For this review, take the finished solid that the model builds, in its own axes (mm). Face numbers are marked on the shaded views. Give positions to 0.01 mm unless a question says otherwise; leave off trailing zeros. Loops run counter-clockwise (first coordinate to the right, second up) from the corner with the lowest first, then second, coordinate; pieces in that order, holes last. Notation, with made-up numbers: (-21, 45.5) -> (2, 45.5) arc R25 cw to (2, 68.5) -> close; hole circle Ø7 at (43, -38). An arc over 180 degrees is marked (long way). Answer as CSV lines item,"result". Start each with the question number.
Item 1: Add section A-A on z = 11.5. State the section outline as (x, y) points.
Item 2: Add section C-C on x = 2.5. State the section outline as (y, z) points.
Item 3: Clearance check with flat-ended pins moving along their axes: P1, Ø4, axis at y = -5, z = 9.5, coming from the +X side; P2, Ø3, axis at x = 16, y = -5, coming from the +Z side; P3, Ø3.5, axis at x = 10, y = -5, coming from the -Z side. State where each tip first meets the part, or that it passes through.
Item 4: The part is to be moulded in two halves that separate along Z. For the marked faces 1 and 2, say which applies: +Z half, -Z half, draft (parallel to the pull), parting line (faces both ways), or undercut.
Item 5: For L1, parallel to Z at x = 11, y = -0.8; L2, parallel to Z at x = 5.75, y = -6.25; L3, parallel to Y at x = 19, z = 20.5, list the stretches that pass through material, from the lowest coordinate up. Write a range as from..to.
Item 6: Add section D-D on y = -2.5. State the section outline as (x, z) points.
Item 7: Add section B-B on x = 11. State how many separate pieces and enclosed holes the cut face has, plus the area to 3 significant figures.
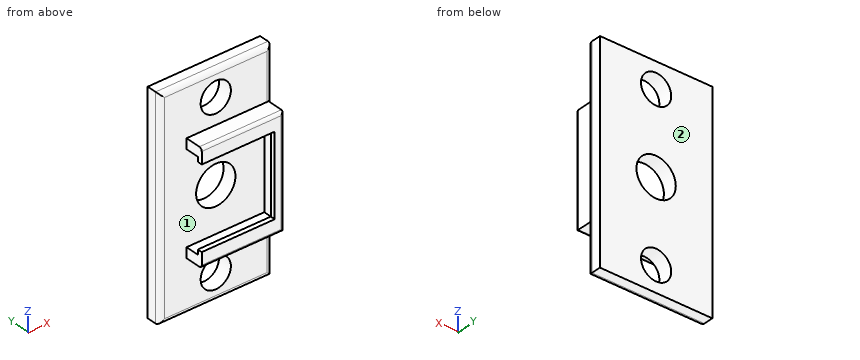
```python
from build123d import *

# Parameters (mm, degrees)
F1_DEPTH      = 3
F2_DEPTH      = 6.85
F6_DEPTH      = 3
F3_W          = 16.2
F3_H          = 1
F7_DEPTH      = 1
F5_W          = 16.2
F5_H          = 1
F8_DEPTH      = 1
F4_W          = 1
F4_H          = 18.8
F9_DEPTH      = 1
F10_D         = 8.2
F0_W          = 23.4142135624
F0_H          = 44.4142135624
F11_DEPTH     = 3
F12_T1_DEPTH  = 28.4142135624
F12_T3_DEPTH  = 49.4142135624
F12_T8_DEPTH  = 49.4142135624
F12_T14_DEPTH = 49.4142135624
F12_T20_DEPTH = 49.4142135624
F12_T27_DEPTH = 49.4142135624
F12_T33_DEPTH = 49.4142135624
F13_R         = 0.6
F14_D         = 6.3


# Not quite as in the source:
# - a fillet or chamfer that OpenCascade refuses, or shapes differently, is made with other operations: its cross-section is extruded or revolved along the edge and cut away or added
# - a feature names something its author has since deleted; it is built from what else it names


with BuildPart() as f1:
    # F0 (on Front) → F1 (new body)
    with BuildSketch(Plane.XZ):
        Polygon((0.9, 2.1), (4.9, 2.1), (21.1, 2.1), (21.1, 20.9), (4.9, 20.9), (0.9, 20.9), align=None)
        Polygon((0, 23), (0, 0), (4.9, 0), (4.9, 2.1), (0.9, 2.1), (0.9, 20.9), (4.9, 20.9), (4.9, 23), align=None)
        Polygon((4.9, 2.1), (4.9, 0), (22, 0), (22, 23), (4.9, 23), (4.9, 20.9), (21.1, 20.9), (21.1, 2.1), align=None)
    extrude(amount=F1_DEPTH)

    # F0 (on Front) → F2 (join)
    with BuildSketch(Plane.XZ):
        Polygon((4.9, 2.1), (4.9, 0), (22, 0), (22, 23), (4.9, 23), (4.9, 20.9), (21.1, 20.9), (21.1, 2.1), align=None)
    extrude(amount=F2_DEPTH)

    # F0 (on Front) → F6 (join)
    with BuildSketch(Plane.XZ):
        Polygon((0, 23), (0, 0), (4.9, 0), (4.9, 2.1), (0.9, 2.1), (0.9, 20.9), (4.9, 20.9), (4.9, 23), align=None)
    extrude(amount=F6_DEPTH)

    # F3 (on face) → F7 (join)
    with BuildSketch(Plane(origin=(0, 0, 20.9), x_dir=(1, 0, 0), z_dir=(0, 0, -1))):
        with Locations((13, 6.35)):
            Rectangle(F3_W, F3_H)
    extrude(amount=F7_DEPTH)

    # F5 (on face) → F8 (join)
    with BuildSketch(Plane.XY.offset(2.1)):
        with Locations((13, -6.35)):
            Rectangle(F5_W, F5_H)
    extrude(amount=F8_DEPTH)

    # F4 (on face) → F9 (join)
    with BuildSketch(Plane(origin=(21.1, 0, 0), x_dir=(0, -1, 0), z_dir=(-1, 0, 0))):
        with Locations((6.35, 11.5)):
            Rectangle(F4_W, F4_H)
    extrude(amount=F9_DEPTH)

    # F10 (through all)
    with Locations(Plane(origin=(0, 0, 0), x_dir=(1, 0, 0), z_dir=(0, 1, 0))):
        with Locations((11, -11.5)):
            Hole(F10_D / 2)

    # F0 (on Front) → F11 (join)
    with BuildSketch(Plane.XZ):
        with Locations((11, 11.5)):
            Rectangle(F0_W, F0_H)
        Polygon((4.9, 0), (0, 0), (0, 23), (4.9, 23), (22, 23), (22, 0), align=None, mode=Mode.SUBTRACT)
    extrude(amount=F11_DEPTH)

    # F12: fillet of radius 1 on 4 edges, made by hand

    # F12_s2 → F12_t1 (cut)
    with BuildSketch(Plane.YZ.offset(-3.2071067812)):
        with BuildLine():
            ThreePointArc((-3, -9.7071067812), (-2.7071067812, -10.4142135624), (-2, -10.7071067812))
            Line((-2, -10.7071067812), (-3, -10.7071067812))
            Line((-3, -10.7071067812), (-3, -9.7071067812))
        make_face()
        with BuildLine():
            ThreePointArc((-3, 32.7071067812), (-2.7071067812, 33.4142135624), (-2, 33.7071067812))
            Line((-2, 33.7071067812), (-3, 33.7071067812))
            Line((-3, 33.7071067812), (-3, 32.7071067812))
        make_face()
    extrude(amount=F12_T1_DEPTH, mode=Mode.SUBTRACT)

    # F12_s4 → F12_t3 (cut)
    with BuildSketch(Plane.XY.offset(-13.2071067812)):
        with BuildLine():
            ThreePointArc((0.2928932188, -3), (-0.4142135624, -2.7071067812), (-0.7071067812, -2))
            Line((-0.7071067812, -2), (-0.7071067812, -3))
            Line((-0.7071067812, -3), (0.2928932188, -3))
        make_face()
    extrude(amount=F12_T3_DEPTH, mode=Mode.SUBTRACT)


with BuildPart() as f12_tool6:
    # F12_s7 → F12_t8 (new body)
    with BuildSketch(Plane.XY.offset(-13.2071067812)):
        with BuildLine():
            ThreePointArc((21.7071067812, -3), (22.4142135624, -2.7071067812), (22.7071067812, -2))
            Line((22.7071067812, -2), (22.7071067812, -3))
            Line((22.7071067812, -3), (21.7071067812, -3))
        make_face()
    extrude(amount=F12_T8_DEPTH)

    split(bisect_by=Plane.XY, keep=Keep.BOTTOM)

    split(bisect_by=Plane.YZ.offset(22), keep=Keep.BOTTOM)


with BuildPart() as f1_1:
    add(f1.part)

    # F12_t5: cut F12_tool6
    add(f12_tool6.part, mode=Mode.SUBTRACT)


with BuildPart() as f12_tool12:
    # F12_s13 → F12_t14 (new body)
    with BuildSketch(Plane.XY.offset(-13.2071067812)):
        with BuildLine():
            ThreePointArc((21.7071067812, -3), (22.4142135624, -2.7071067812), (22.7071067812, -2))
            Line((22.7071067812, -2), (22.7071067812, -3))
            Line((22.7071067812, -3), (21.7071067812, -3))
        make_face()
    extrude(amount=F12_T14_DEPTH)

    split(bisect_by=Plane.XY, keep=Keep.BOTTOM)

    split(bisect_by=Plane.YZ.offset(22), keep=Keep.TOP)


with BuildPart() as f1_2:
    add(f1_1.part)

    # F12_t11: cut F12_tool12
    add(f12_tool12.part, mode=Mode.SUBTRACT)


with BuildPart() as f12_tool18:
    # F12_s19 → F12_t20 (new body)
    with BuildSketch(Plane.XY.offset(-13.2071067812)):
        with BuildLine():
            ThreePointArc((21.7071067812, -3), (22.4142135624, -2.7071067812), (22.7071067812, -2))
            Line((22.7071067812, -2), (22.7071067812, -3))
            Line((22.7071067812, -3), (21.7071067812, -3))
        make_face()
    extrude(amount=F12_T20_DEPTH)

    split(bisect_by=Plane.XY.offset(23), keep=Keep.BOTTOM)

    split(bisect_by=Plane.XY, keep=Keep.TOP)

    split(bisect_by=Plane.YZ.offset(22), keep=Keep.TOP)


with BuildPart() as f1_3:
    add(f1_2.part)

    # F12_t17: cut F12_tool18
    add(f12_tool18.part, mode=Mode.SUBTRACT)


with BuildPart() as f12_tool25:
    # F12_s26 → F12_t27 (new body)
    with BuildSketch(Plane.XY.offset(-13.2071067812)):
        with BuildLine():
            ThreePointArc((21.7071067812, -3), (22.4142135624, -2.7071067812), (22.7071067812, -2))
            Line((22.7071067812, -2), (22.7071067812, -3))
            Line((22.7071067812, -3), (21.7071067812, -3))
        make_face()
    extrude(amount=F12_T27_DEPTH)

    split(bisect_by=Plane.XY.offset(23), keep=Keep.TOP)

    split(bisect_by=Plane.YZ.offset(22), keep=Keep.BOTTOM)


with BuildPart() as f1_4:
    add(f1_3.part)

    # F12_t24: cut F12_tool25
    add(f12_tool25.part, mode=Mode.SUBTRACT)


with BuildPart() as f12_tool31:
    # F12_s32 → F12_t33 (new body)
    with BuildSketch(Plane.XY.offset(-13.2071067812)):
        with BuildLine():
            ThreePointArc((21.7071067812, -3), (22.4142135624, -2.7071067812), (22.7071067812, -2))
            Line((22.7071067812, -2), (22.7071067812, -3))
            Line((22.7071067812, -3), (21.7071067812, -3))
        make_face()
    extrude(amount=F12_T33_DEPTH)

    split(bisect_by=Plane.XY.offset(23), keep=Keep.TOP)

    split(bisect_by=Plane.YZ.offset(22), keep=Keep.TOP)


with BuildPart() as f1_5:
    add(f1_4.part)

    # F12_t30: cut F12_tool31
    add(f12_tool31.part, mode=Mode.SUBTRACT)

    # F13
    f13_edges = [f1_5.edges().sort_by_distance(p)[0] for p in [
        (22, -6.85, 11.5),
        (13.45, -6.85, 0),
        (13.45, -6.85, 23),
    ]]
    fillet(f13_edges, radius=F13_R)

    # F14 (through all)
    with Locations(Plane(origin=(0, 0, 0), x_dir=(1, 0, 0), z_dir=(0, 1, 0))):
        with Locations((11, -28.3535533906), (11, 5.3535533906)):
            Hole(F14_D / 2)


solid = f1_5.part
```
Computed values:
1,outline,"(-0.71, -2) arc R1 ccw to (0.29, -3) -> (6.9, -3) -> (6.9, 0) -> (-0.71, 0) -> close; (15.1, -3) -> (21.1, -3) -> (21.1, -5.85) -> (20.1, -5.85) -> (20.1, -6.85) -> (21.4, -6.85) arc R0.6 ccw to (22, -6.25) -> (22, -2.96) arc R1 ccw to (22.71, -2) -> (22.71, 0) -> (15.1, 0) -> close"
2,outline,"(-3, -9.71) arc R1 ccw to (-2, -10.71) -> (0, -10.71) -> (0, 33.71) -> (-2, 33.71) arc R1 ccw to (-3, 32.71) -> close"
3,P1,"x = 22"
3,P2,"z = 23"
3,P3,"z = 0"
4,face 1,"undercut"
4,face 2,"draft"
5,L1,"-10.71..-8.5, -2.2..7.4, 15.6..25.2, 31.5..33.71"
5,L2,"0..3.1, 19.9..23"
5,L3,"-6.85..-5.85, -3..0"
6,outline,"(-0.57, -10.57) -> (22.57, -10.57) -> (22.57, 33.57) -> (-0.57, 33.57) -> close; hole circle Ø8.2 at (11, 11.5); hole circle Ø6.3 at (11, -5.35); hole circle Ø6.3 at (11, 28.35)"
7,separate pieces,"4"
7,enclosed holes,"0"
7,area,"88.4 mm²"
